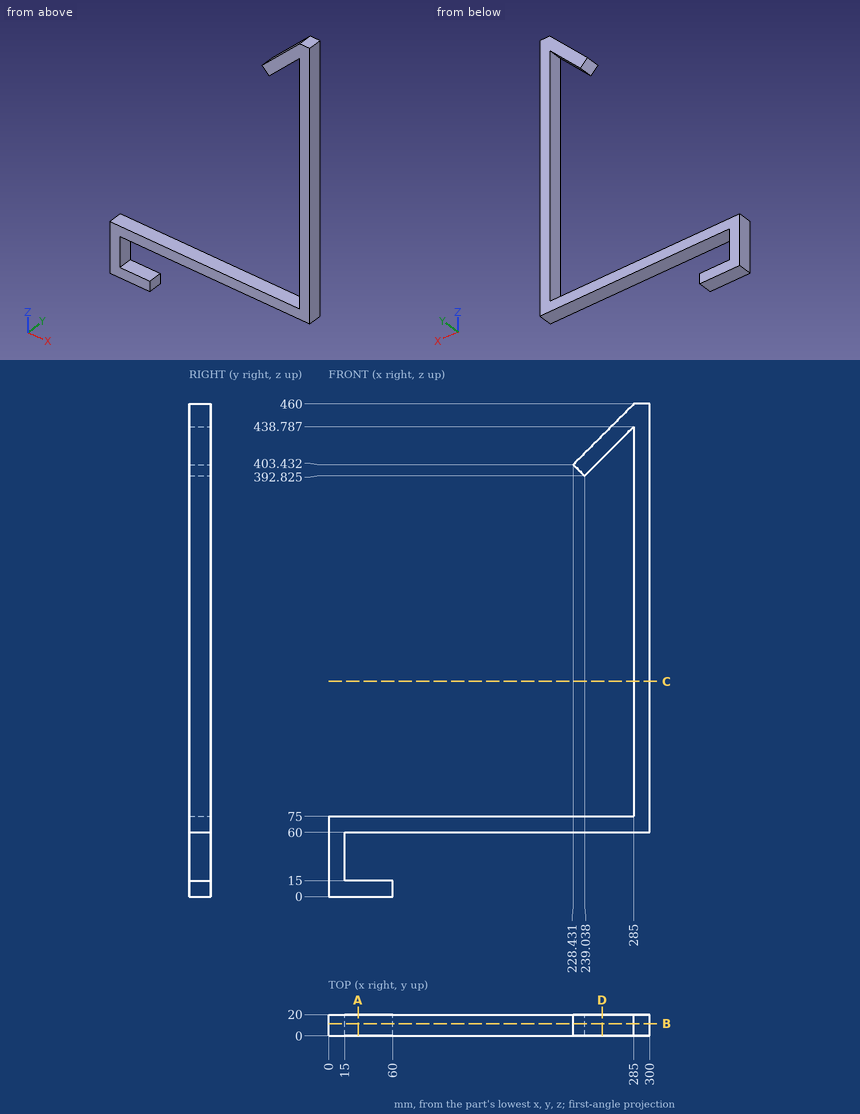
Study the drawing (mm; zero at the part's minimum x, y, z) and answer. Coordinates: 2 decimals unless noted, no trailing zeros. Write each loop counter-clockwise with the first axis right and the second up, starting at its lowest first coordinate (ties: lowest second). Pieces come first, ordered by that corner, then holes. Notation, with made-up numbers: (7, 4) - (27, 4) arc R26 cw to (27, 32) - close; hole circle Ø7 at (73, -1.5). An arc over 180 degrees is marked (long way). Answer as a JSON object with one key per item and string values. Group by question number.
1. A cutting plane is placed at D-D (x = 255.5). Determine the outline of the cut face in (y, z), plus the area to 3 significant figures.
2. A cutting plane is placed at C-C (z = 201). Determine the outline of the cut face in (x, y), plus the area to 3 significant figures.
3. A cutting plane is placed at B-B (y = 11.5). Determine the outline of the cut face in (x, z) (1 decimal).
4. Each of these flat-tipped pins is pushed along its axis until it touches: P1, Ø4.5, axis at y = 14.5, z = 7.5, coming from the +X side; P2, Ø8, axis at x = 102.5, y = 12.5, coming from the +Z side; P3, Ø6, axis at y = 8, z = 29.5, coming from the +X side. Where does it stop, or does it pass through?
5. Consider L1, parallel to Z at x = 59, y = 13.5; L2, parallel to X at y = 12.25, z = 328; L3, parallel to Z at x = 212, y = 16.75. Determine where each line is inside the solid, lowest interval first. Write a range as [from, to].
6. A cutting plane is placed at A-A (x = 27.5). Determine the outline of the cut face in (y, z).
Worked out:
{
 "1": {"outline": "(0, 60) - (20, 60) - (20, 75) - (0, 75) - close; (0, 409.29) - (20, 409.29) - (20, 430.5) - (0, 430.5) - close", "area": "724 mm²"},
 "2": {"outline": "(285, 0) - (300, 0) - (300, 20) - (285, 20) - close", "area": "300 mm²"},
 "3": {"outline": "(0, 0) - (60, 0) - (60, 15) - (15, 15) - (15, 60) - (300, 60) - (300, 460) - (285, 460) - (228.4, 403.4) - (239, 392.8) - (285, 438.8) - (285, 75) - (0, 75) - close"},
 "4": {"P1": "stops at x = 60", "P2": "stops at z = 75", "P3": "stops at x = 15"},
 "5": {"L1": "z = [0, 15], [60, 75]", "L2": "x = [285, 300]", "L3": "z = [60, 75]"},
 "6": {"outline": "(0, 0) - (20, 0) - (20, 15) - (0, 15) - close; (0, 60) - (20, 60) - (20, 75) - (0, 75) - close"}
}
